from build123d import *

# Parameters (mm, degrees)
F0_R     = 37.5
F1_DEPTH = 152.6
F2_T     = -3
F4_R     = 39
F4_R_2   = 37.5
F5_DEPTH = 5


with BuildPart() as f1:
    # F0 (on Top) → F1 (new body)
    with BuildSketch(Plane.XY):
        Circle(F0_R)
    extrude(amount=F1_DEPTH)

    # F2
    f2_openings = [f1.faces().sort_by_distance(p)[0] for p in [
        (0, 0, 152.6),
        (0, 0, 0),
    ]]
    offset(amount=F2_T, openings=f2_openings)

    # F4 (on Top) → F5 (join)
    with BuildSketch(Plane.XY):
        Circle(F4_R)
        Circle(F4_R_2, mode=Mode.SUBTRACT)
    extrude(amount=F5_DEPTH)


solid = f1.part
Model file for the job. Use its own axes, mm. A direction names the side the tool comes from. Give positions to 0.01 mm unless a question says otherwise; leave off trailing zeros. Loops run counter-clockwise (first coordinate to the right, second up) from the corner with the lowest first, then second, coordinate; pieces in that order, holes last. Notation, with made-up numbers: (59.25, 44) -> (91.25, 44) arc R11 ccw to (91.25, 50) -> close; hole circle Ø10 at (18.5, 67.5). An arc over 180 degrees is marked (long way). Use a Markdown table: item, result. Add a question column.
(1) Wall check: line 1 along X through (y, z) = (1, 48); line 2 along Y through (x, z) = (0, 50); line 3 along X through (y, z) = (-22, 14). Give the ranges that are in metal, low to high.
(2) Tool access for faces 1 (the flat face through (-20, 32, 5)), 2 (the cylindrical face through (-5.077, 38.668, 2.465)): list every direction of +Z, -Z, +X, -X, +Y, -Y with a clear straight run to the whole face (end or side of a thin tool).
(3) Slice it at A-A on y = 0. List the corners of the cut face in (x, z).
(4) Drop flat-ended pins along their axis: pin 1 Ø6 at (y, z) = (-21.5, 115) entering from -X; pin 2 Ø12 at (x, z) = (-12, 130) entering from +Y; pin 3 Ø4 at (x, z) = (6.5, 17.5) entering from -Y. Give the stop position or say it passes through.
(5) Slice it at C-C on z = 10.5. List the corners of the cut face in (x, y).
(6) Mould opens along X. For faces 3 (the cylindrical face through (32.907, 10.363, 75.232)), 4 (the cylindrical face through (-4.88, 37.18, 77.77)), 5 (the flat face through (11, -33, 152.6)) say: +X half, -X half, draft (parallel to the pull), parting line (faces both ways), or undercut.
Filled sheet:
| question | item | result |
|---|---|---|
| 1 | line 1 | -37.49 to -34.49, 34.49 to 37.49 |
| 1 | line 2 | -37.5 to -34.5, 34.5 to 37.5 |
| 1 | line 3 | -30.37 to -26.58, 26.58 to 30.37 |
| 2 | face 1 | +Z |
| 2 | face 2 | +Z, -Z |
| 3 | outline | (-39, 0) -> (-34.5, 0) -> (-34.5, 152.6) -> (-37.5, 152.6) -> (-37.5, 5) -> (-39, 5) -> close; (34.5, 0) -> (39, 0) -> (39, 5) -> (37.5, 5) -> (37.5, 152.6) -> (34.5, 152.6) -> close |
| 4 | pin 1 | x = -32.62 |
| 4 | pin 2 | y = 37.02 |
| 4 | pin 3 | y = -37.23 |
| 5 | outline | circle Ø75 at (0, 0); hole circle Ø69 at (0, 0) |
| 6 | face 3 | undercut |
| 6 | face 4 | parting line |
| 6 | face 5 | draft |
